Build history of the part. All positions in model axes, mm. Face numbers are marked on the shaded views. Round coordinates to 2 decimals unless told otherwise and drop trailing zeros. Loops run counter-clockwise (first coordinate to the right, second up) from the corner with the lowest first, then second, coordinate; pieces in that order, holes last. Notation, with made-up numbers: (38, 6.25) - (90, 6.25) arc R26 ccw to (90, 26.25) - close; hole circle Ø5 at (11.5, -4.75). An arc over 180 degrees is marked (long way). Use one line per item in the form item = value. Start each with the question number.
Q1. Saw through at C-C (x = 13). Give the cut face in (y, z) (3 decimals).
Q2. Pin check, flat tips, straight feed: pin 1 (10 mm diameter, centred on x = 15.5, z = -6.5, fed in from +Y); pin 2 (5 mm diameter, centred on y = -16.5, z = 0.5, fed in from +X); pin 3 (4 mm diameter, centred on y = -5, z = -5, fed in from -X); pin 4 (5.5 mm diameter, centred on x = 16.764, y = -22.225, fed in from -Z) (3 decimals). Stop position of each tip, or through.
Q3. Saw through at A-A (x = 0). Count the separate pieces of the cut face and the enclosed holes in it, then the cut area to 3 significant figures.
Q4. Drill centre lines: line 1 (Y direction, x = -15.5, z = 7.75); line 2 (Y direction, x = 16, z = 4); line 3 (Y direction, x = -13, z = 3.5). Where is each one in solid material? Low to high.
Q5. Saw through at B-B (y = 0). Give the cut face in (x, z) (3 decimals).
Q6. Mould opens along Y. For the marked faces 1, 2 and 3 say: released by +Y, released by -Y, zero draft, split by the parting line, or undercut.
```python
from build123d import *

# Parameters (mm, degrees)
F0_R     = 31.75
F0_R_2   = 2.0955
F0_R_3   = 23.5
F1_DEPTH = 9.525


with BuildPart() as f1:
    # F0 (on Top) → F1 (new body, symmetric)
    with BuildSketch(Plane.XY):
        Circle(F0_R)
        with Locations((-16.764, -22.225)):
            Circle(F0_R_2, mode=Mode.SUBTRACT)
        with Locations((16.764, -22.225)):
            Circle(F0_R_2, mode=Mode.SUBTRACT)
        Circle(F0_R_3, mode=Mode.SUBTRACT)
        with Locations((0, 27.686)):
            Circle(F0_R_2, mode=Mode.SUBTRACT)
    extrude(amount=F1_DEPTH, both=True)


solid = f1.part
```
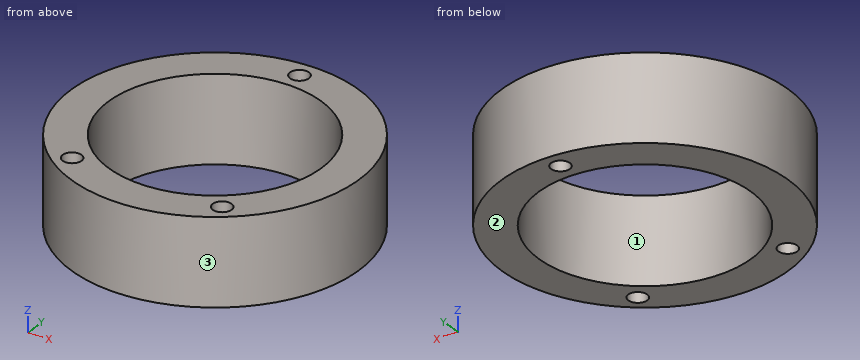
Report:
q1.outline = (-28.967, -9.525) - (-19.577, -9.525) - (-19.577, 9.525) - (-28.967, 9.525) - close; (19.577, -9.525) - (28.967, -9.525) - (28.967, 9.525) - (19.577, 9.525) - close
q2.pin_1 = 29.96
q2.pin_2 = 28.5
q2.pin_3 = -31.61
q2.pin_4 = -9.525
q3.separate_pieces = 3
q3.enclosed_holes = 0
q3.area = 234 mm²
q4.line_1 = -27.71 to -23.9, -20.55 to -17.66, 17.66 to 27.71
q4.line_2 = -27.42 to -24.18, -20.27 to -17.21, 17.21 to 27.42
q4.line_3 = -28.97 to -19.58, 19.58 to 28.97
q5.outline = (-31.75, -9.525) - (-23.5, -9.525) - (-23.5, 9.525) - (-31.75, 9.525) - close; (23.5, -9.525) - (31.75, -9.525) - (31.75, 9.525) - (23.5, 9.525) - close
q6.face_1 = undercut
q6.face_2 = zero draft
q6.face_3 = split by the parting line
